from build123d import *

# Parameters (mm, degrees)
F4_DEPTH = 102.616


# Not quite as in the source:
# - a feature of the source that left no trace in its solid (it failed there, or was rolled back) is left out


with BuildPart() as f4:
    # F3 (on Top) → F4 (new body)
    with BuildSketch(Plane.XY):
        with BuildLine():
            Line((-116.903886199, 40.9632176161), (-116.903886199, 37.3379997909))
            add(Edge.make_bspline(
                [(-116.903886199, 37.3379997909), (-94.3898521159, 11.5008250837), (-44.1040481936, -46.2073180434), (-101.1608146078, -129.3041537381), (-132.6720416546, -175.1967519522)],
                knots=[0, 0, 0, 0, 0.4477214706, 1, 1, 1, 1], degree=3))
            add(Edge.make_bspline(
                [(-138.4897381067, -196.8956440687), (-136.550505956, -189.6626800299), (-134.6112738053, -182.429715991), (-132.6720416546, -175.1967519522)],
                knots=[0, 0, 0, 0, 22.4652511914, 22.4652511914, 22.4652511914, 22.4652511914], degree=3))
            add(Edge.make_bspline(
                [(-68.5538262124, 40.9632176161), (-60.3988212358, 13.7210225854), (-40.7807645704, -51.8140601445), (-102.453603187, -143.3879738574), (-138.4897381067, -196.8956440687)],
                knots=[0, 0, 0, 0, 0.4156887257, 1, 1, 1, 1], degree=3))
            Line((-68.5538262124, 40.9632176161), (-116.903886199, 40.9632176161))
        make_face()
        Polygon((-88.0872011185, 3.8100015372), (-107.6205760246, 37.6427993178), (-68.5538262124, 37.6427993178), align=None, mode=Mode.SUBTRACT)
    extrude(amount=F4_DEPTH)


solid = f4.part
Source: CAD feature listing. Evaluate the final solid. Frame: model axes, mm. A direction names the side the tool comes from. Coordinates: 2 decimals unless noted, no trailing zeros. Return JSON: item names as keys, results as strings.
Q1. Access query for faces 1 (the flat face through (-68, -51, 0)), 2 (the flat face through (-97.717, 20.49, 50.59)). Directions: +Z, -Z, +X, -X, +Y, -Y. A direction counts if a zero-diameter tool reaches every point of the face in a straight line with its end or side. Return the directions, or none.
Results:
{"face 1": "-Z, +X, -X, +Y, -Y", "face 2": "+Z, -Z"}
Q2. Section A-A, the plane x = -78. Give the number of separate pieces and of enclosed holes in the cut face, plus the area to 3 significant figures.
Results:
{"separate pieces": "3", "enclosed holes": "0", "area": "5,960 mm2"}
Q3. Contact query for flat-ended pins moving along their axis: P1, Ø12, axis at x = -128, z = 67, coming from the +Y side; P2, Ø10, axis at y = -33.5, z = 62.5, coming from the -X side; P3, Ø4, axis at y = -47, z = 28.5, coming from the -X side. Output: stop coordinate, or through.
Results:
{"P1": "y = -159.6", "P2": "x = -73.53", "P3": "x = -70.89"}
Q4. Material intervals for line 1 along Y through (x, z) = (-85, 71); line 2 along Y through (x, z) = (-81.5, 68.5); line 3 along Y through (x, z) = (-70.5, 97), sorted ascending.
Results:
{"line 1": "-112.56 to -98.46, -3.37 to 9.16, 37.64 to 40.96", "line 2": "-106.09 to -90.85, -9.39 to 15.22, 37.64 to 40.96", "line 3": "-83.48 to 34.27, 37.64 to 40.96"}
Q5. Mould query, pull axis X, two halves, no side actions, for faces 3 (the flat face through (-68, -51, 102.616)), 4 (the flat face through (-78.184, 20.963, 50.59)). Classes: released by +X, released by -X, zero draft, split by the parting line, or undercut.
Results:
{"face 3": "zero draft", "face 4": "undercut"}
